from build123d import *

# Parameters (mm, degrees)
CYLINDER027_R          = 1.7
CYLINDER027_DEPTH      = 10.5
CYLINDER026_R          = 1.7
CYLINDER026_DEPTH      = 11.5
CYLINDER018_R          = 26.7
CYLINDER018_DEPTH      = 30
CYLINDER019_R          = 28
CYLINDER019_DEPTH      = 30
FILLET001_R            = 1
BOX001_W               = 8
BOX001_H               = 13.5
BOX001_DEPTH           = 20
BOX001_PLACEMENT_ANGLE = 237
FILLET004_1_R          = 2.5
FILLET004_2_R          = 2
CYLINDER021_R          = 3
CYLINDER021_DEPTH      = 5.5
CYLINDER020_R          = 3
CYLINDER020_DEPTH      = 5.5
BOX_W                  = 8
BOX_H                  = 13.5
BOX_DEPTH              = 20
BOX_PLACEMENT_ANGLE    = 51
FILLET003_1_R          = 2.5
FILLET003_2_R          = 2


with BuildPart() as obj1:
    # Cylinder027 → Cylinder027 (new body)
    with BuildSketch(Plane(origin=(2.2, 8, -3.4), x_dir=(1, 0, 0), z_dir=(0, 0, 1))):
        Circle(CYLINDER027_R)
    extrude(amount=CYLINDER027_DEPTH)


with BuildPart() as obj2:
    # Cylinder026 → Cylinder026 (new body)
    with BuildSketch(Plane(origin=(-29.1, 29.1, -3.4), x_dir=(1, 0, 0), z_dir=(0, 0, 1))):
        Circle(CYLINDER026_R)
    extrude(amount=CYLINDER026_DEPTH)

    # Fusion007: union obj1
    add(obj1.part)


with BuildPart() as base_exterior_vaciado001:
    # Cylinder018 → Cylinder018 (new body)
    with BuildSketch(Plane(origin=(-12.5, 19, -10.6), x_dir=(1, 0, 0), z_dir=(0, 0, 1))):
        Circle(CYLINDER018_R)
    extrude(amount=CYLINDER018_DEPTH)


with BuildPart() as base:
    # Cylinder019 → Cylinder019 (new body)
    with BuildSketch(Plane(origin=(-12.5, 19, -10), x_dir=(1, 0, 0), z_dir=(0, 0, 1))):
        Circle(CYLINDER019_R)
    extrude(amount=CYLINDER019_DEPTH)

    # Cut011: cut base exterior vaciado001
    add(base_exterior_vaciado001.part, mode=Mode.SUBTRACT)

    # Fillet001
    fillet001_edges = [base.edges().sort_by_distance(p)[0] for p in [
        (-40.5, 19, 20),
        (-39.2, 19, 19.4),
    ]]
    fillet(fillet001_edges, radius=FILLET001_R)


with BuildPart() as obj3:
    # Box001 → Box001 (new body)
    with BuildSketch(Plane.XY):
        with Locations((4, 6.75)):
            Rectangle(BOX001_W, BOX001_H)
    extrude(amount=BOX001_DEPTH)


with BuildPart() as obj3_1:
    # Box001 placement: moved
    add(obj3.part.moved(Location((-33.471804, 36.855151, 0))).rotate(Axis((-33.471804, 36.855151, 0), (0, 0, 1)), BOX001_PLACEMENT_ANGLE))

    # Fillet004 1
    fillet004_1_edges = [obj3_1.edges().sort_by_distance(p)[0] for p in [
        (-35.65036, 33.500468, 20),
    ]]
    fillet(fillet004_1_edges, radius=FILLET004_1_R)

    # Fillet004 2
    fillet004_2_edges = [obj3_1.edges().sort_by_distance(p)[0] for p in [
        (-22.149751, 29.502524, 10),
        (-26.506863, 22.793159, 10),
    ]]
    fillet(fillet004_2_edges, radius=FILLET004_2_R)


with BuildPart() as obj4:
    # Cylinder021 → Cylinder021 (new body)
    with BuildSketch(Plane(origin=(-29.1, 29.1, -1.8), x_dir=(1, 0, 0), z_dir=(0, 0, 1))):
        Circle(CYLINDER021_R)
    extrude(amount=CYLINDER021_DEPTH)


with BuildPart() as obj5:
    # Cylinder020 → Cylinder020 (new body)
    with BuildSketch(Plane(origin=(2.2, 8, -1.8), x_dir=(1, 0, 0), z_dir=(0, 0, 1))):
        Circle(CYLINDER020_R)
    extrude(amount=CYLINDER020_DEPTH)


with BuildPart() as base_v10_final:
    # Box → Box (new body)
    with BuildSketch(Plane.XY):
        with Locations((4, 6.75)):
            Rectangle(BOX_W, BOX_H)
    extrude(amount=BOX_DEPTH)


with BuildPart() as base_v10_final_1:
    # Box placement: moved
    add(base_v10_final.part.moved(Location((6.739128, -1.032332, 0))).rotate(Axis((6.739128, -1.032332, 0), (0, 0, 1)), BOX_PLACEMENT_ANGLE))

    # Fillet003 1
    fillet003_1_edges = [base_v10_final_1.edges().sort_by_distance(p)[0] for p in [
        (9.256409, 2.076252, 20),
    ]]
    fillet(fillet003_1_edges, radius=FILLET003_1_R)

    # Fillet003 2
    fillet003_2_edges = [base_v10_final_1.edges().sort_by_distance(p)[0] for p in [
        (-3.752343, 7.463494, 10),
        (1.282221, 13.680661, 10),
    ]]
    fillet(fillet003_2_edges, radius=FILLET003_2_R)

    # Fusion006: union base, obj3, obj4, obj5
    add(base.part)
    add(obj3_1.part)
    add(obj4.part)
    add(obj5.part)

    # Cut019: cut obj2
    add(obj2.part, mode=Mode.SUBTRACT)


solid = base_v10_final_1.part
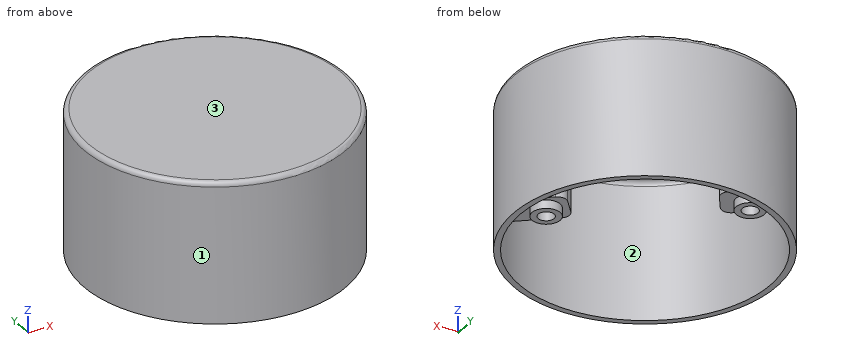
Input: part model. Units: mm. Frame: model coordinates. Face numbers are marked on the shaded views. Coordinates: 2 decimals unless noted, no trailing zeros. Loops run counter-clockwise (first coordinate to the right, second up) from the corner with the lowest first, then second, coordinate; pieces in that order, holes last.
Q1. Cut plane C-C (y = 19). Output: boundary loops of the cut face in (x, z), then the cut area to 3 significant figures.
Q2. Cut plane A-A (z = 16). Output: boundary loops of the cut face in (x, y), then the cut area to 3 significant figures.
Q3. Contact query for flat-ended pins moving along their axis: pin 1 (2 mm diameter, centred on x = -26.5, y = 23.5, fed in from -Z); pin 2 (10 mm diameter, centred on x = -19, z = 14, fed in from +Y); pin 3 (1 mm diameter, centred on y = 35, z = -2, fed in from +X). Output: stop coordinate, or through.
Q4. Cut plane D-D (z = -2.5). Output: boundary loops of the cut face in (x, y), then the cut area to 3 significant figures.
Q5. Material intervals for line 1 (X direction, y = 8, z = 4.25); line 2 (X direction, y = 29, z = 3); line 3 (Y direction, x = 1, z = 4.5), sorted ascending.
Q6. Cut plane B-B (x = -12.5). Output: boundary loops of the cut face in (y, z).
Q7. Draft query along X for the marked faces 1, 2 and 3. Return one class per face: +X half, -X half, draft (parallel to the pull), parting line (faces both ways), or undercut.
Working result:
1. outline: (-40.5, -10) - (-39.2, -10) - (-39.2, 18.4) arc R1 cw to (-38.2, 19.4) - (13.2, 19.4) arc R1 cw to (14.2, 18.4) - (14.2, -10) - (15.5, -10) - (15.5, 19) arc R1 ccw to (14.5, 20) - (-39.5, 20) arc R1 ccw to (-40.5, 19) - close
1. area: 110 mm2
2. outline: circle Ø56 at (-12.5, 19); hole (-37, 29.61) arc R26.7 ccw to (5.9, -0.35) - (-2.2, 6.2) arc R2 cw to (-2.49, 9.02) - (0.02, 12.13) arc R2 cw to (2.84, 12.42) - (10.8, 5.97) arc R26.7 ccw to (-32.76, 36.39) - (-23.83, 30.59) arc R2 cw to (-23.24, 27.83) - (-25.42, 24.47) arc R2 cw to (-28.18, 23.88) - close
2. area: 423 mm2
3. pin 1: stops at z = 0
3. pin 2: stops at y = 46.96
3. pin 3: stops at x = 10.82
4. outline: circle Ø56 at (-12.5, 19); hole circle Ø53.4 at (-12.5, 19)
4. area: 223 mm2
5. line 1: x = -38.25 to -36.83, -2.92 to 0.5, 3.9 to 8.3, 11.83 to 13.25
5. line 2: x = -38.65 to -37.26, -36.06 to -30.8, -27.4 to -22.92, 12.26 to 13.65
5. line 3: y = -5.53 to -4.04, 3.62 to 6.8, 9.2 to 12.78, 42.04 to 43.53
6. outline: (-9, -10) - (-7.7, -10) - (-7.7, 18.4) arc R1 cw to (-6.7, 19.4) - (44.7, 19.4) arc R1 cw to (45.7, 18.4) - (45.7, -10) - (47, -10) - (47, 19) arc R1 ccw to (46, 20) - (-8, 20) arc R1 ccw to (-9, 19) - close
7. face 1: parting line
7. face 2: undercut
7. face 3: draft
